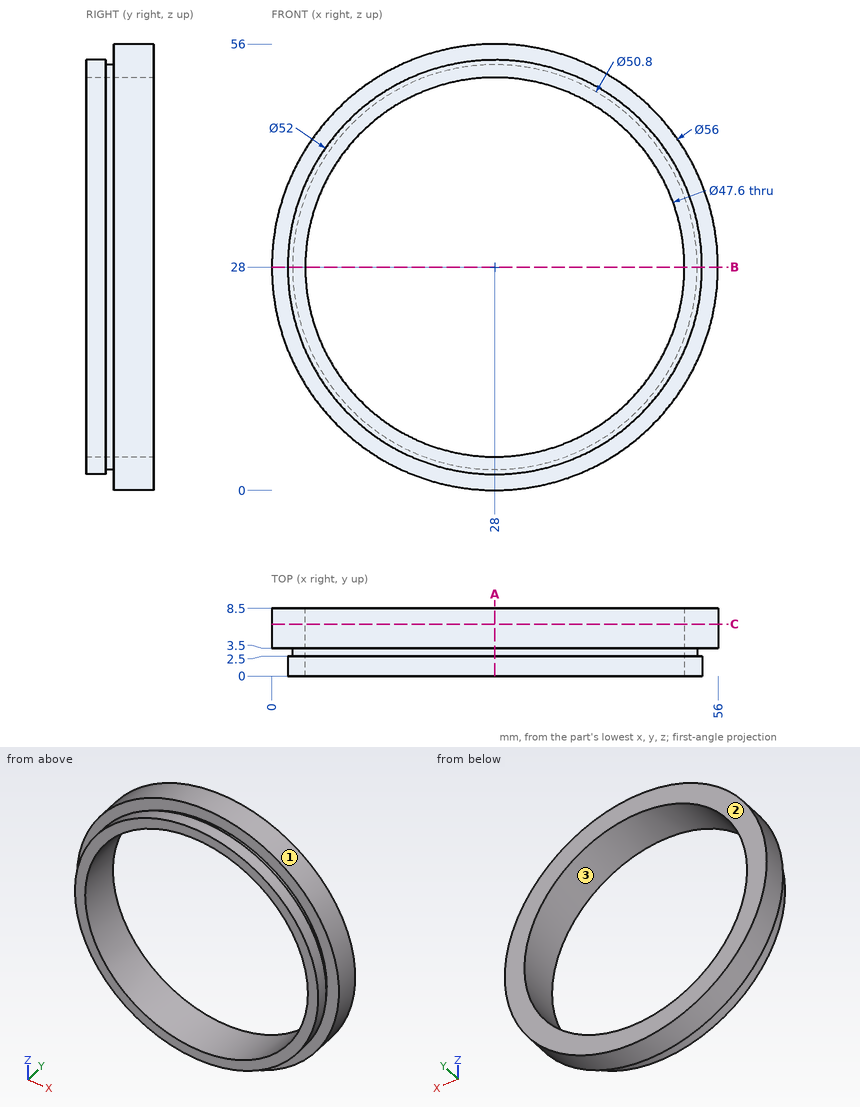
Study the drawing (mm; zero at the part's minimum x, y, z) and answer. Round coordinates to 2 decimals unless told otherwise and drop trailing zeros. Loops run counter-clockwise (first coordinate to the right, second up) from the corner with the lowest first, then second, coordinate; pieces in that order, holes last. Notation, with made-up numbers: (53, 38.5) -> (89, 38.5) arc R6 ccw to (89, 49.5) -> close; hole circle Ø6 at (-35.5, 51). An arc over 180 degrees is marked (long way). Use one line per item in the form item = value.
1. The part is cut by section C-C on y = 6.5. Determine the outline of the cut face in (x, z).
Answer key:
outline = circle Ø56 at (28, 28); hole circle Ø47.6 at (28, 28)
2. The part is cut by section A-A on x = 28. Determine the outline of the cut face in (y, z).
Answer key:
outline = (0, 2) -> (2.5, 2) -> (2.5, 2.6) -> (3.5, 2.6) -> (3.5, 0) -> (8.5, 0) -> (8.5, 4.2) -> (0, 4.2) -> close; (0, 51.8) -> (8.5, 51.8) -> (8.5, 56) -> (3.5, 56) -> (3.5, 53.4) -> (2.5, 53.4) -> (2.5, 54) -> (0, 54) -> close
3. Flat-ended cylindrical pins translate along their axes: pin 1 Ø3 at (y, z) = (1, 28.5) entering from +X; pin 2 Ø1 at (y, z) = (5, 9.5) entering from +X; pin 3 Ø3 at (x, y) = (50, 6) entering from -Z. Find the tip coordinate at first contact, or state that the pin passes through.
Answer key:
pin_1 = 54
pin_2 = 49.45
pin_3 = 8.93
4. The part is cut by section B-B on z = 28. Determine the outline of the cut face in (x, y).
Answer key:
outline = (0, 3.5) -> (2.6, 3.5) -> (2.6, 2.5) -> (2, 2.5) -> (2, 0) -> (4.2, 0) -> (4.2, 8.5) -> (0, 8.5) -> close; (51.8, 0) -> (54, 0) -> (54, 2.5) -> (53.4, 2.5) -> (53.4, 3.5) -> (56, 3.5) -> (56, 8.5) -> (51.8, 8.5) -> close
5. Find the intervals of material crossed by probe 1 along Z at (x, y) = (28, 3.25); probe 2 along Y at (x, z) = (51.5, 39); probe 3 along Z at (x, y) = (28, 6.5), in increasing order. Write a range as [from, to].
Answer key:
probe_1 = [2.6, 4.2], [51.8, 53.4]
probe_2 = [0, 2.5], [3.5, 8.5]
probe_3 = [0, 4.2], [51.8, 56]
6. For a pull along X with two mould halves and no side action, classify the marked faces 1, 2 and 3 as released by +X, released by -X, zero draft, split by the parting line, or undercut.
Answer key:
face_1 = split by the parting line
face_2 = zero draft
face_3 = undercut
